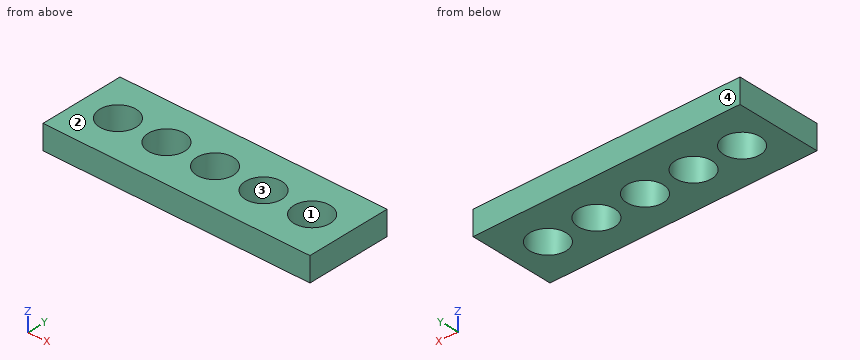
from build123d import *

# Parameters (mm, degrees)
CYLINDER_R     = 1.5
CYLINDER_DEPTH = 5
ARRAY_X_COUNT  = 5
ARRAY_X_PITCH  = 4
BOX_W          = 22
BOX_H          = 7
BOX_DEPTH      = 2


with BuildPart() as array:
    # Cylinder → Cylinder (new body)
    with BuildSketch(Plane.XY):
        Circle(CYLINDER_R)
    extrude(amount=CYLINDER_DEPTH)

    # Array X: Array ×5


with BuildPart() as array_1:
    add(array.part)
    with Locations(*[(i * ARRAY_X_PITCH, 0, 0) for i in range(1, ARRAY_X_COUNT)]):
        add(array.part)


with BuildPart() as cut:
    # Box → Box (new body)
    with BuildSketch(Plane(origin=(-3, -3.5, 2), x_dir=(1, 0, 0), z_dir=(0, 0, 1))):
        with Locations((11, 3.5)):
            Rectangle(BOX_W, BOX_H)
    extrude(amount=BOX_DEPTH)

    # Cut: cut Array
    add(array_1.part, mode=Mode.SUBTRACT)


solid = cut.part
The listing builds one solid part. Answer for the finished solid, in the listing's coordinates (mm). Face numbers are marked on the shaded views. Coordinates: 2 decimals unless noted, no trailing zeros. Order: outer loops, then holes, each group sorted by start corner. A loop starts at its lowest first (then second) coordinate and runs counter-clockwise, first axis right, second up. Notation, with made-up numbers: (26, 57.25) -> (48, 57.25) arc R16 ccw to (48, 73.25) -> close; hole circle Ø11 at (-4, 3.25). An arc over 180 degrees is marked (long way). Answer in a Markdown table with one row per item. Add a question column.
Item 1: Find the intervals of material crossed by L1, parallel to X at y = 0, z = 3.2; L2, parallel to Y at x = 8, z = 2.45; L3, parallel to X at y = 1, z = 2.85, in increasing order. Write a range as from..to.
Item 2: Determine the mould class of the marked faces 1, 2, 3 and 4 for opening direction Y: +Y half, -Y half, draft (parallel to the pull), parting line (faces both ways), or undercut.
Item 3: Find section B-B (z = 2.7). Write down the section's boundary in (x, y).
Item 4: Find section C-C (x = 4). Write down the section's boundary in (y, z), then the cut area to 3 significant figures.
Item 5: Find section D-D (x = 15). Write down the section's boundary in (y, z).
Item 6: Find section A-A (y = 0). Write down the section's boundary in (x, z).
Result set:
| question | item | result |
|---|---|---|
| 1 | L1 | x = -3..-1.5, 1.5..2.5, 5.5..6.5, 9.5..10.5, 13.5..14.5, 17.5..19 |
| 1 | L2 | y = -3.5..-1.5, 1.5..3.5 |
| 1 | L3 | x = -3..-1.12, 1.12..2.88, 5.12..6.88, 9.12..10.88, 13.12..14.88, 17.12..19 |
| 2 | face 1 | undercut |
| 2 | face 2 | draft |
| 2 | face 3 | undercut |
| 2 | face 4 | +Y half |
| 3 | outline | (-3, -3.5) -> (19, -3.5) -> (19, 3.5) -> (-3, 3.5) -> close; hole circle Ø3 at (0, 0); hole circle Ø3 at (4, 0); hole circle Ø3 at (8, 0); hole circle Ø3 at (12, 0); hole circle Ø3 at (16, 0) |
| 4 | outline | (-3.5, 2) -> (-1.5, 2) -> (-1.5, 4) -> (-3.5, 4) -> close; (1.5, 2) -> (3.5, 2) -> (3.5, 4) -> (1.5, 4) -> close |
| 4 | area | 8.00 mm² |
| 5 | outline | (-3.5, 2) -> (-1.12, 2) -> (-1.12, 4) -> (-3.5, 4) -> close; (1.12, 2) -> (3.5, 2) -> (3.5, 4) -> (1.12, 4) -> close |
| 6 | outline | (-3, 2) -> (-1.5, 2) -> (-1.5, 4) -> (-3, 4) -> close; (1.5, 2) -> (2.5, 2) -> (2.5, 4) -> (1.5, 4) -> close; (5.5, 2) -> (6.5, 2) -> (6.5, 4) -> (5.5, 4) -> close; (9.5, 2) -> (10.5, 2) -> (10.5, 4) -> (9.5, 4) -> close; (13.5, 2) -> (14.5, 2) -> (14.5, 4) -> (13.5, 4) -> close; (17.5, 2) -> (19, 2) -> (19, 4) -> (17.5, 4) -> close |
